Job drawing, mm, ordinate dimensions from the low corner. One solid piece. A direction names the side the tool comes from. Round coordinates to 2 decimals unless told otherwise and drop trailing zeros. Write each loop counter-clockwise with the first axis right and the second up, starting at its lowest first coordinate (ties: lowest second). Pieces come first, ordered by that corner, then holes. Notation, with made-up numbers: (38.5, -1) -> (44.5, -1) arc R25 cw to (44.5, 26) -> close; hole circle Ø8 at (81.5, 83). An arc over 180 degrees is marked (long way). Use CSV: the item, a comma, the result in double quotes. Start each with the question number.
(1) Probe line 1 (X direction, y = 1.65, z = 7.5); line 2 (Y direction, x = 17, z = 2.5) (3 decimals); line 3 (X direction, y = 0.75, z = 6.75). List the from-to ranges inside material, lowest first. Write a range as [from, to].
(2) Which spindle directions (+Z, -Z, +X, -X, +Y, -Y) get a long thin tool onto all of the face, cutting with end or side? Do the marked faces 5 and 6. Say none if no direction does.
(3) Saw through at D-D (x = 15). Give the cut face in (y, z) (3 decimals).
(4) Saw through at C-C (y = 2). Give the cut face in (x, z).
(5) Drop flat-ended pins along their axis: pin 1 (1.5 mm diameter, centred on x = 15.5, y = 6.5, fed in from +Z); pin 2 (1 mm diameter, centred on x = 6.5, z = 5, fed in from +Y) (3 decimals); pin 3 (1.5 mm diameter, centred on y = 6.5, z = 3.5, fed in from +X). Give the stop position or say it passes through.
(6) Saw through at B-B (x = 5). Give the cut face in (y, z) (3 decimals), plus the area to 3 significant figures.
(7) Two-plate mould, pull along X, no slides. Class the marked faces 1, 2, 3 and 4: released by +X, released by -X, zero draft, split by the parting line, or undercut.
(8) Saw through at A-A (z = 7.5). Give the cut face in (x, y) (3 decimals).
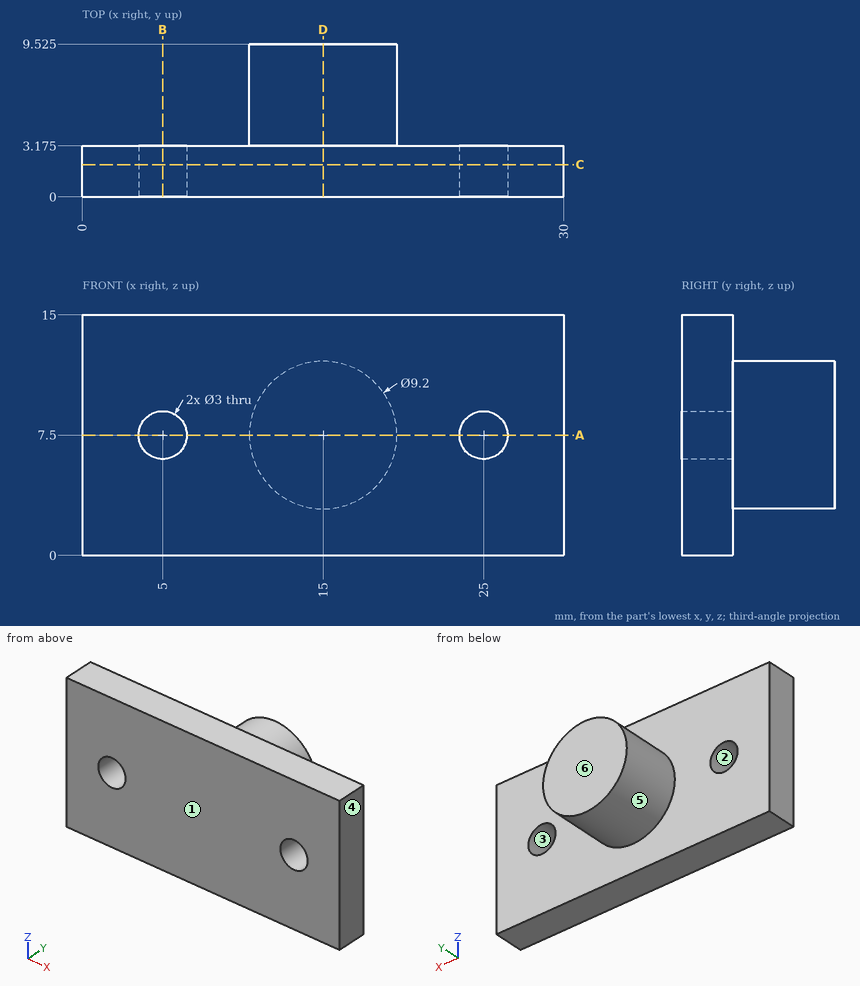
Answers:
1,line 1,"x = [0, 3.5], [6.5, 23.5], [26.5, 30]"
1,line 2,"y = [0, 3.175]"
1,line 3,"x = [0, 3.7], [6.3, 23.7], [26.3, 30]"
2,face 5,"+Y"
2,face 6,"+Z, -Z, +X, -X, +Y"
3,outline,"(0, 0) -> (3.175, 0) -> (3.175, 2.9) -> (9.525, 2.9) -> (9.525, 12.1) -> (3.175, 12.1) -> (3.175, 15) -> (0, 15) -> close"
4,outline,"(0, 0) -> (30, 0) -> (30, 15) -> (0, 15) -> close; hole circle Ø3 at (5, 7.5); hole circle Ø3 at (25, 7.5)"
5,pin 1,"stops at z = 12.1"
5,pin 2,"stops at y = 3.175"
5,pin 3,"stops at x = 18.26"
6,outline,"(0, 0) -> (3.175, 0) -> (3.175, 6) -> (0, 6) -> close; (0, 9) -> (3.175, 9) -> (3.175, 15) -> (0, 15) -> close"
6,area,"38.1 mm²"
7,face 1,"zero draft"
7,face 2,"undercut"
7,face 3,"undercut"
7,face 4,"released by +X"
8,outline,"(0, 0) -> (3.5, 0) -> (3.5, 3.175) -> (0, 3.175) -> close; (6.5, 0) -> (23.5, 0) -> (23.5, 3.175) -> (19.6, 3.175) -> (19.6, 9.525) -> (10.4, 9.525) -> (10.4, 3.175) -> (6.5, 3.175) -> close; (26.5, 0) -> (30, 0) -> (30, 3.175) -> (26.5, 3.175) -> close"
